Here's how the part is built. I have some questions about the finished solid (model axes, mm). Round coordinates to 2 decimals unless told otherwise and drop trailing zeros. Order: outer loops, then holes, each group sorted by start corner. A loop starts at its lowest first (then second) coordinate and runs counter-clockwise, first axis right, second up. Notation, with made-up numbers: (72, -1.5) - (92, -1.5) arc R12 cw to (92, 19.5) - close; hole circle Ø5 at (85.5, 12.5). An arc over 180 degrees is marked (long way). One line per item, written item: value.
from build123d import *

# Parameters (mm, degrees)
F0_W     = 152.4
F0_H     = 6.35
F2_W     = 1.5875
F2_H     = 14.605
F3_DEPTH = 25.4
F4_COUNT = 6


with BuildPart() as f1:
    # F0 (on Top) → F1 (revolve)
    with BuildSketch(Plane.XY):
        with Locations((76.2, 3.175)):
            Rectangle(F0_W, F0_H)
    revolve(axis=Axis((76.2, 0, 0), (1, 0, 0)))

    # F2 (on face) → F3 (join)
    with BuildSketch(Plane(origin=(0, 0, 0), x_dir=(0, -1, 0), z_dir=(-1, 0, 0))):
        Rectangle(F2_W, F2_H)
    extrude(amount=-F3_DEPTH)

    # F4: F1 ×6 about axis
    f4_axis = Axis((152.4, 0, 0), (-1, 0, 0))


with BuildPart() as f1_1:
    add(f1.part)
    for i in range(1, F4_COUNT):
        add(f1.part.rotate(f4_axis, i * 360 / F4_COUNT))


solid = f1_1.part
Q1. If we section it at B-B, the plane z = 0: Please give me the cut outline in (x, y).
Results list:
outline: (0, -6.35) - (152.4, -6.35) - (152.4, 6.35) - (0, 6.35) - close
Q2. If I drill on line 1 along Z through (x, y) = (59, 0.5); line 2 along Z through (x, y) = (20, 2.5); line 3 along Y through (x, z) = (83.5, -4), over which ranges is the centre line in solid material (lowest first)?
Results list:
line 1: -6.33 to 6.33
line 2: -5.84 to 5.84
line 3: -4.93 to 4.93
Q3. Will these pins go through, and if not, where does the flat tip stop? pin 1 (2 mm diameter, centred on x = 78.5, y = -4.5, fed in from +Z); pin 2 (0.5 mm diameter, centred on y = -6, z = 3, fed in from +X); pin 3 (6 mm diameter, centred on x = 31, z = 2.5, fed in from -Y).
Results list:
pin 1: z = 5.3
pin 2: x = 25.4
pin 3: y = -6.35
Q4. If we section it at C-C, the plane x = 68: Please give me the cut outline in (y, z), then the cut area to 3 significant figures.
Results list:
outline: circle Ø12.7 at (0, 0)
area: 127 mm²
Q5. If we section it at A-A, the plane x = 18: Please give me the cut outline in (y, z), then the cut area to 3 significant figures.
Results list:
outline: (-6.72, -2.96) - (-5.93, -4.34) - (-5.06, -3.84) arc R6.35 ccw to (-0.79, -6.3) - (-0.79, -7.3) - (0.79, -7.3) - (0.79, -6.3) arc R6.35 ccw to (5.06, -3.84) - (5.93, -4.34) - (6.72, -2.96) - (5.85, -2.46) arc R6.35 ccw to (5.85, 2.46) - (6.72, 2.96) - (5.93, 4.34) - (5.06, 3.84) arc R6.35 ccw to (0.79, 6.3) - (0.79, 7.3) - (-0.79, 7.3) - (-0.79, 6.3) arc R6.35 ccw to (-5.06, 3.84) - (-5.93, 4.34) - (-6.72, 2.96) - (-5.85, 2.46) arc R6.35 ccw to (-5.85, -2.46) - close
area: 136 mm²
